from build123d import *

# Parameters (mm, degrees)
EXTRUDE_1_DEPTH      = 3.5
EXTRUDE_1_DEPTH_BACK = 5.5
SKETCH_1_R           = 6
SKETCH_2_W           = 14.3
SKETCH_2_H           = 11.3
EXTRUDE_2_DEPTH      = 13
SKETCH_3_R           = 1.25
EXTRUDE_3_DEPTH      = 1
SKETCH_4_R           = 4.75
EXTRUDE_4_DEPTH      = 11.5
SKETCH_5_R           = 4.25
CUT_EXTRUDE_1_DEPTH  = 11.5


with BuildPart() as part:
    # 草圖1 → 填料-伸長1 (new, two sides: drawn at the far end of the back side and taken through both)
    with BuildSketch(Plane.XY.offset(-EXTRUDE_1_DEPTH_BACK)):
        with Locations((-64.340909091, 31.5)):
            Circle(SKETCH_1_R)
    extrude(amount=EXTRUDE_1_DEPTH + EXTRUDE_1_DEPTH_BACK)

    # 草圖2 → 填料-伸長2 (add)
    with BuildSketch(Plane.XY.offset(3.5)):
        with Locations((-64.340909091, 31.2)):
            Rectangle(SKETCH_2_W, SKETCH_2_H)
    extrude(amount=EXTRUDE_2_DEPTH)

    # 草圖3 → 填料-伸長3 (add)
    with BuildSketch(Plane.XZ.offset(-25.55)):
        with BuildLine():
            Line((-50.690909091, 7.087920564), (-79.690909091, 7.087920564))
            ThreePointArc((-79.690909091, 7.087920564), (-80.751569263, 7.527260393), (-81.190909091, 8.587920564))
            Line((-81.190909091, 8.587920564), (-81.190909091, 48.087920564))
            ThreePointArc((-81.190909091, 48.087920564), (-80.751569263, 49.148580736), (-79.690909091, 49.587920564))
            Line((-79.690909091, 49.587920564), (-50.690909091, 49.587920564))
            ThreePointArc((-50.690909091, 49.587920564), (-49.630248919, 49.148580736), (-49.190909091, 48.087920564))
            Line((-49.190909091, 48.087920564), (-49.190909091, 8.587920564))
            ThreePointArc((-49.190909091, 8.587920564), (-49.630248919, 7.527260393), (-50.690909091, 7.087920564))
        make_face()
        with Locations(Location((-51.190909091, 47.587920564, 0), (0, 0, 270))):
            Circle(SKETCH_3_R, mode=Mode.SUBTRACT)
        with Locations(Location((-79.190909091, 47.587920564, 0), (0, 0, 270))):
            Circle(SKETCH_3_R, mode=Mode.SUBTRACT)
    extrude(amount=EXTRUDE_3_DEPTH)

    # 草圖4 → 填料-伸長4 (add)
    with BuildSketch(Plane(origin=(0, 0, -5.5), x_dir=(-1, 0, 0), z_dir=(0, 0, -1))):
        with Locations((64.340909091, 31.5)):
            Circle(SKETCH_4_R)
    extrude(amount=EXTRUDE_4_DEPTH)

    # 草圖5 → 除料-伸長1 (cut)
    with BuildSketch(Plane(origin=(0, 0, -17), x_dir=(-1, 0, 0), z_dir=(0, 0, -1))):
        with Locations((64.340909091, 31.5)):
            Circle(SKETCH_5_R)
    extrude(amount=-CUT_EXTRUDE_1_DEPTH, mode=Mode.SUBTRACT)


solid = part.part
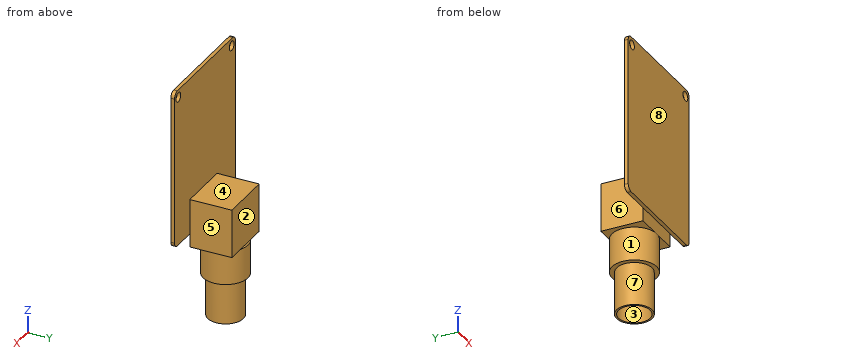
Could you check a few things on this model? Use its own coordinates, in mm. Face numbers are marked on the shaded views. A direction names the side the tool comes from. Give positions to 0.01 mm unless a question says otherwise; leave off trailing zeros. Loops run counter-clockwise (first coordinate to the right, second up) from the corner with the lowest first, then second, coordinate; pieces in that order, holes last. Notation, with made-up numbers: (-5.75, 45.25) -> (45.25, 45.25) arc R35 ccw to (45.25, 82.25) -> close; hole circle Ø6 at (52.25, 55). An arc over 180 degrees is marked (long way). Answer as CSV lines item,"result". Start each with the question number.
(1) I'm going to push flat-ended pins straight in: pin 1 Ø5.5 at (x, y) = (-65, 32.5) entering from +Z; pin 2 Ø6 at (x, z) = (-70.5, 21) entering from +Y; pin 3 Ø3 at (x, z) = (-66, 4.5) entering from -Y. Where does each tip first touch, or does it pass through?
(2) If we section it at A-A on y = 31.5: Write out the boundary of the cut face in (x, z).
(3) If we section it at D-D on x = -73: Write out the boundary of the cut face in (y, z), then the cut area to 3 significant figures.
(4) If we section it at B-B on x = -66: Write out the boundary of the cut face in (y, z).
(5) Which directions (+Z, -Z, +X, -X, +Y, -Y) give clear straight access to the entire face, cutting with the end or side of a thin tool? Please do the marked faces 4, 5, 6, 7 and 8.
(6) We'd pull the mould along X, two halves only. Please class the marked faces 1, 2 and 3: released by +X, released by -X, zero draft, split by the parting line, or undercut.
(7) I need wall thicknesses on probe 1 along Y at (x, z) = (-65.5, 22); probe 2 along X at (y, z) = (31.75, -5); probe 3 along Z at (x, y) = (-61.5, 34.75). Which ranges of each line are inside material? Lowest first, please.
(8) If we section it at C-C on z = 36: Write out the boundary of the cut face in (x, y), then the cut area to 3 significant figures.
Computed:
1,pin 1,"stops at z = 16.5"
1,pin 2,"stops at y = 25.55"
1,pin 3,"stops at y = 25.52"
2,outline,"(-71.49, 3.5) -> (-70.34, 3.5) -> (-70.34, -5.5) -> (-69.09, -5.5) -> (-69.09, -17) -> (-68.59, -17) -> (-68.59, -5.5) -> (-60.09, -5.5) -> (-60.09, -17) -> (-59.59, -17) -> (-59.59, -5.5) -> (-58.34, -5.5) -> (-58.34, 3.5) -> (-57.19, 3.5) -> (-57.19, 16.5) -> (-71.49, 16.5) -> close"
3,outline,"(24.55, 7.09) -> (25.55, 7.09) -> (25.55, 49.59) -> (24.55, 49.59) -> close"
3,area,"42.5 mm2"
4,outline,"(24.55, 7.09) -> (25.55, 7.09) -> (25.55, 3.5) -> (25.73, 3.5) -> (25.73, -5.5) -> (27.05, -5.5) -> (27.05, -17) -> (27.59, -17) -> (27.59, -5.5) -> (35.41, -5.5) -> (35.41, -17) -> (35.95, -17) -> (35.95, -5.5) -> (37.27, -5.5) -> (37.27, 3.5) -> (36.85, 3.5) -> (36.85, 16.5) -> (25.55, 16.5) -> (25.55, 49.59) -> (24.55, 49.59) -> close"
5,face 4,"+Z, +X, -X, +Y"
5,face 5,"+Z, -Z, +X, +Y"
5,face 6,"+Z, -Z, -X, +Y"
5,face 7,"-Z"
5,face 8,"+Z, -Z, +X, -X, -Y"
6,face 1,"split by the parting line"
6,face 2,"zero draft"
6,face 3,"undercut"
7,probe 1,"y = 24.55 to 25.55"
7,probe 2,"x = -70.34 to -58.35"
7,probe 3,"z = -17 to 16.5"
8,outline,"(-81.19, 24.55) -> (-49.19, 24.55) -> (-49.19, 25.55) -> (-81.19, 25.55) -> close"
8,area,"32.0 mm2"
